For this review, take the finished solid that the model builds, in its own axes (mm). Face numbers are marked on the shaded views. A direction names the side the tool comes from. Give positions to 0.01 mm unless a question says otherwise; leave off trailing zeros. Write each loop counter-clockwise with the first axis right and the second up, starting at its lowest first coordinate (ties: lowest second). Pieces come first, ordered by that corner, then holes. Notation, with made-up numbers: (-35, -15.75) -> (9, -15.75) arc R4 cw to (9, -11.75) -> close; hole circle Ø5 at (24, 0). An arc over 180 degrees is marked (long way). Answer as CSV lines item,"result".
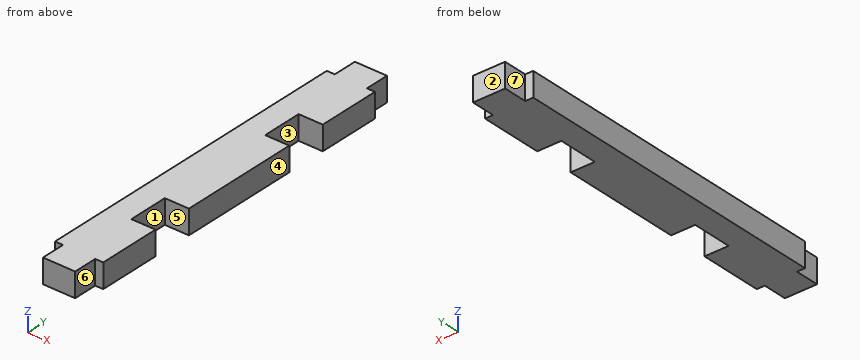
Autodesk Inventor part; units mm, degrees
ref_plane "YZ Plane" through (0, 0, 0) normal (1, 0, 0) x (0, 1, 0)
ref_plane "XZ Plane" through (0, 0, 0) normal (0, 1, 0) x (-1, 0, 0)
ref_plane "XY Plane" through (0, 0, 0) normal (0, 0, 1) x (1, 0, 0)
sketch "Sketch1" plane through (0, 0, 0) normal (0, 0, 1) x (1, 0, 0)
  line L0 (-3, 20.3) -> (3, 20.3)
  line L1 (3, 20.3) -> (3, -20.3)
  line L2 (3, -20.3) -> (-3, -20.3)
  line L3 (-3, -20.3) -> (-3, 20.3)
  line L4 (-2, -20.3) -> (2, -20.3)
  line L5 (2, -20.3) -> (2, -23.3)
  line L6 (2, -23.3) -> (-2, -23.3)
  line L7 (-2, -23.3) -> (-2, -20.3)
  line L8 (-2, 20.3) -> (2, 20.3)
  line L9 (2, 20.3) -> (2, 23.3)
  line L10 (2, 23.3) -> (-2, 23.3)
  line L11 (-2, 23.3) -> (-2, 20.3)
  line L12 (3, -12.5) -> (0, -12.5)
  line L13 (0, -12.5) -> (0, -7.5)
  line L14 (0, -7.5) -> (3, -7.5)
  line L15 (3, -7.5) -> (3, -12.5)
  line L16 (3, 7.5) -> (0, 7.5)
  line L17 (0, 7.5) -> (0, 12.5)
  line L18 (0, 12.5) -> (3, 12.5)
  line L19 (3, 12.5) -> (3, 7.5)
  point P0 (0, 0)
  point P1 (0, 23.3)
  point P2 (0, 20.3)
  point P3 (0, 20.3)
  point P4 (0, -23.3)
  point P5 (3, 0)
  point P6 (3, -10)
  point P7 (3, 10)
  dimension "d0" = 46.6
  dimension "d1" = 3
  dimension "d2" = 4
  dimension "d3" = 6
  dimension "d6" = 5
  dimension "d7" = 10
  dimension "d8" = 10
  dimension "d9" = 3
extrude "Extrusion1" add sketch "Sketch1" along normal blind 3 contours L0 L1 L18 L17 L16 L14 L13 L12 L2 L3 | L11 L10 L9 L0 | L2 L5 L6 L7
properties material "MDF Medium Density Fiberboard"
Q1. Draft analysis for pull direction Y (two halves, no side actions). For the marked faces 1, 2, 3 and 4, state which applies: released by +Y, released by -Y, zero draft, split by the parting line, or undercut.
Answer block:
face 1,"undercut"
face 2,"released by +Y"
face 3,"undercut"
face 4,"zero draft"
Q2. Clearance check with flat-ended pins moving along their axes: pin 1 (0.5 mm diameter, centred on x = 2.5, z = 1, fed in from +Y); pin 2 (0.5 mm diameter, centred on x = -2.5, z = 2, fed in from -Y); pin 3 (0.9 mm diameter, centred on y = 21.5, z = 2, fed in from +X). State where each tip first meets the part, or that it passes through.
Answer block:
pin 1,"stops at y = 20.3"
pin 2,"stops at y = -20.3"
pin 3,"stops at x = 2"
Q3. Add section C-C (y = -10.5). Write out the cut boundary in (x, z).
Answer block:
outline,"(-3, 0) -> (0, 0) -> (0, 3) -> (-3, 3) -> close"
Q4. For the marked faces 5, 6 and 7, list the 3-axis set-ups (+Z, -Z, +X, -X, +Y, -Y) from which the entire face can be reached by the end or side of a thin tool; tool diameter is ignored.
Answer block:
face 5,"+Z, -Z, +X"
face 6,"+Z, -Z, +X, -Y"
face 7,"+Z, -Z, -X, +Y"
Q5. Add section A-A (x = 0.7). Write out the cut boundary in (y, z), plus the area to 3 significant figures.
Answer block:
outline,"(-23.3, 0) -> (-12.5, 0) -> (-12.5, 3) -> (-23.3, 3) -> close; (-7.5, 0) -> (7.5, 0) -> (7.5, 3) -> (-7.5, 3) -> close; (12.5, 0) -> (23.3, 0) -> (23.3, 3) -> (12.5, 3) -> close"
area,"110 mm2"
Q6. Add section B-B (z = 0.45). Write out the cut boundary in (x, y), plus the area to 3 significant figures.
Answer block:
outline,"(-3, -20.3) -> (-2, -20.3) -> (-2, -23.3) -> (2, -23.3) -> (2, -20.3) -> (3, -20.3) -> (3, -12.5) -> (0, -12.5) -> (0, -7.5) -> (3, -7.5) -> (3, 7.5) -> (0, 7.5) -> (0, 12.5) -> (3, 12.5) -> (3, 20.3) -> (2, 20.3) -> (2, 23.3) -> (-2, 23.3) -> (-2, 20.3) -> (-3, 20.3) -> close"
area,"238 mm2"
Q7. To check wall thickness, follow probe 1 along Y at (x, z) = (1, 1); probe 2 along Y at (x, z) = (2.7, 0.8); probe 3 along X at (y, z) = (11, 1.1). State the ranges of each line that lie inside material, in increasing order. Write a range as [from, to].
Answer block:
probe 1,"y = [-23.3, -12.5], [-7.5, 7.5], [12.5, 23.3]"
probe 2,"y = [-20.3, -12.5], [-7.5, 7.5], [12.5, 20.3]"
probe 3,"x = [-3, 0]"
